Read the model definition and answer for the solid it produces. Units are mm, in the model's axes. A direction names the side the tool comes from. Coordinates: 2 decimals unless noted, no trailing zeros. Loops run counter-clockwise (first coordinate to the right, second up) from the corner with the lowest first, then second, coordinate; pieces in that order, holes last. Notation, with made-up numbers: M 17.25,53 L 70.25,53 A24 ccw 70.25,79 Z; hole C 73.5,78.5 d6. An arc over 180 degrees is marked long. One line per item, written item: value. Start each with the question number.
```python
from build123d import *

# Parameters (mm, degrees)
SKETCH_1_W          = 35
SKETCH_1_H          = 21
EXTRUDE_1_DEPTH     = 20
SKETCH_2_R          = 5
CUT_EXTRUDE_1_DEPTH = 18
SKETCH_3_W          = 7.5
SKETCH_3_H          = 4
CUT_EXTRUDE_2_DEPTH = 18
FILLET_1_R          = 0.5
SKETCH_7_W          = 8
SKETCH_7_H          = 13
CUT_EXTRUDE_3_DEPTH = 29.574464124
FILLET_2_R          = 1
SKETCH_8_R          = 1.5
CUT_EXTRUDE_4_DEPTH = 34.871079109


with BuildPart() as part:
    # 草图1 → 凸台-拉伸1 (new body)
    with BuildSketch(Plane.XY):
        Rectangle(SKETCH_1_W, SKETCH_1_H)
    extrude(amount=EXTRUDE_1_DEPTH)

    # 草图2 → 切除-拉伸1 (cut)
    with BuildSketch(Plane.XY.offset(20)):
        Circle(SKETCH_2_R)
    extrude(amount=-CUT_EXTRUDE_1_DEPTH, mode=Mode.SUBTRACT)

    # 草图3 → 切除-拉伸2 (cut)
    with BuildSketch(Plane.XY.offset(20)):
        with Locations((-3.75, 0)):
            Rectangle(SKETCH_3_W, SKETCH_3_H)
    extrude(amount=-CUT_EXTRUDE_2_DEPTH, mode=Mode.SUBTRACT)

    # 圆角1
    fillet_1_edges = [part.edges().sort_by_distance(p)[0] for p in [
        (-7.5, 2, 11),
        (-7.5, -2, 11),
    ]]
    fillet(fillet_1_edges, radius=FILLET_1_R)

    # 草图7 → 切除-拉伸3 (cut, through all)
    with BuildSketch(Plane.XY.offset(20)):
        with Locations((-13.5, 0)):
            Rectangle(SKETCH_7_W, SKETCH_7_H)
        with Locations((13.5, 0)):
            Rectangle(SKETCH_7_W, SKETCH_7_H)
    extrude(amount=-CUT_EXTRUDE_3_DEPTH, mode=Mode.SUBTRACT)

    # 圆角2
    fillet_2_edges = [part.edges().sort_by_distance(p)[0] for p in [
        (-9.5, 6.5, 10),
        (-9.5, -6.5, 10),
        (9.5, 6.5, 10),
        (9.5, -6.5, 10),
    ]]
    fillet(fillet_2_edges, radius=FILLET_2_R)

    # 草图8 → 切除-拉伸4 (cut, through all)
    with BuildSketch(Plane(origin=(0, 10.5, 0), x_dir=(1, 0, 0), z_dir=(0, 1, 0))):
        with Locations(Location((-14.5, -4, 0), (0, 0, 270))):
            Circle(SKETCH_8_R)
        with Locations(Location((-14.5, -16, 0), (0, 0, 270))):
            Circle(SKETCH_8_R)
        with Locations(Location((14.5, -16, 0), (0, 0, 270))):
            Circle(SKETCH_8_R)
        with Locations(Location((14.5, -4, 0), (0, 0, 270))):
            Circle(SKETCH_8_R)
    extrude(amount=-CUT_EXTRUDE_4_DEPTH, mode=Mode.SUBTRACT)


solid = part.part
```
1) Section B-B (z = 18) is taken. Determine the outline of the cut face in (x, y), then the cut area to 3 significant figures.
2) Flat-ended cylindrical pins translate along their axes: pin 1 (1.5 mm diameter, centred on y = 0, z = 11.5, fed in from +X); pin 2 (1 mm diameter, centred on y = 5, z = 11.5, fed in from -X). Find the tip coordinate at first contact, or state that the pin passes through.
3) A tool of negligible diameter and unlimited length cuts with its end or side. For faces 1 (the face through (-9.5, 0, 10)), 2 (the face through (9.785, -6.199, 9.86)), 3 (the face through (-6, 2, 11)), from which of +Z, -Z, +X, -X, +Y, -Y can it reach the whole face along a straight path? Write none if from no direction.
4) Section C-C (y = 0) is taken. Determine the outline of the cut face in (x, z).
5) Section D-D (x = 14.5) is taken. Determine the outline of the cut face in (y, z).
6) For a pull along Z with two mould halves and no side action, classify faces 4 (the face through (0, 0, 0)), 5 (the face through (13.925, 8.528, 5.386)), 6 (the face through (-6, -2, 11)) as released by +Z, released by -Z, zero draft, split by the parting line, or undercut.
7) Section A-A (x = -12) is taken. Determine the outline of the cut face in (y, z), then the cut area to 3 significant figures.
8) Consider line 1 along X through (y, z) = (8.1, 16); line 2 along X through (y, z) = (0, 6.75); line 3 along Y through (x, z) = (-13.5, 11.5). Determine where each line is inside the solid, lowest interval first.
Results found:
1. outline: M -17.5,-10.5 L 17.5,-10.5 L 17.5,-6.5 L 10.5,-6.5 A1 cw 9.5,-5.5 L 9.5,5.5 A1 cw 10.5,6.5 L 17.5,6.5 L 17.5,10.5 L -17.5,10.5 L -17.5,6.5 L -10.5,6.5 A1 cw -9.5,5.5 L -9.5,-5.5 A1 cw -10.5,-6.5 L -17.5,-6.5 Z; hole M -7.5,-1.5 A0.5 ccw -7,-2 L -4.58,-2 A5 ccw long -4.58,2 L -7,2 A0.5 ccw -7.5,1.5 Z
1. area: 439 mm²
2. pin 1: stops at x = 9.5
2. pin 2: stops at x = -9.5
3. face 1: +Z, -Z, -X
3. face 2: +Z, -Z, +X
3. face 3: +Z
4. outline: M -9.5,0 L 9.5,0 L 9.5,20 L 5,20 L 5,2 L -7.5,2 L -7.5,20 L -9.5,20 Z
5. outline: M -10.5,0 L -6.5,0 L -6.5,2.5 L -10.5,2.5 Z; M -10.5,5.5 L -6.5,5.5 L -6.5,14.5 L -10.5,14.5 Z; M -10.5,17.5 L -6.5,17.5 L -6.5,20 L -10.5,20 Z; M 6.5,0 L 10.5,0 L 10.5,2.5 L 6.5,2.5 Z; M 6.5,5.5 L 10.5,5.5 L 10.5,14.5 L 6.5,14.5 Z; M 6.5,17.5 L 10.5,17.5 L 10.5,20 L 6.5,20 Z
6. face 4: released by -Z
6. face 5: undercut
6. face 6: zero draft
7. outline: M -10.5,0 L -6.5,0 L -6.5,20 L -10.5,20 Z; M 6.5,0 L 10.5,0 L 10.5,20 L 6.5,20 Z
7. area: 160 mm²
8. line 1: x = -17.5 to -16, -13 to 13, 16 to 17.5
8. line 2: x = -9.5 to -7.5, 5 to 9.5
8. line 3: y = -10.5 to -6.5, 6.5 to 10.5
